```python
from build123d import *

# Parameters (mm, degrees)
SKETCH2_R           = 15
SKETCH2_R_2         = 3
SKETCH2_R_3         = 2.3
BOSS_EXTRUDE1_DEPTH = 4
SKETCH3_R           = 17
SKETCH3_R_2         = 1.475
SKETCH3_R_3         = 1
BOSS_EXTRUDE2_DEPTH = 3
SKETCH8_R           = 15
SKETCH8_R_2         = 12.3
BOSS_EXTRUDE5_DEPTH = 3


with BuildPart() as part:
    # Sketch2 → Boss-Extrude1 (new body)
    with BuildSketch(Plane.XY):
        Circle(SKETCH2_R)
        Circle(SKETCH2_R_2, mode=Mode.SUBTRACT)
        with Locations((-8, 0)):
            Circle(SKETCH2_R_3, mode=Mode.SUBTRACT)
        with Locations((0, 8)):
            Circle(SKETCH2_R_3, mode=Mode.SUBTRACT)
        with Locations((8, 0)):
            Circle(SKETCH2_R_3, mode=Mode.SUBTRACT)
        with Locations((0, -8)):
            Circle(SKETCH2_R_3, mode=Mode.SUBTRACT)
    extrude(amount=BOSS_EXTRUDE1_DEPTH)

    # Sketch3 → Boss-Extrude2 (add)
    with BuildSketch(Plane.XY):
        Circle(SKETCH3_R)
        Circle(SKETCH3_R_2, mode=Mode.SUBTRACT)
        with Locations((-15.8, 0)):
            Circle(SKETCH3_R_3, mode=Mode.SUBTRACT)
        with Locations((15.8, 0)):
            Circle(SKETCH3_R_3, mode=Mode.SUBTRACT)
    extrude(amount=-BOSS_EXTRUDE2_DEPTH)

    # Sketch7 → Cut-Revolve1 (revolve, cut)
    with BuildSketch(Plane(origin=(0, 0, 0), x_dir=(0, 0, -1), z_dir=(1, 0, 0))):
        with BuildLine():
            Line((-4, 15), (0, 15))
            ThreePointArc((0, 15), (-2, 13.505217823), (-4, 15))
        make_face()
    revolve(axis=Axis((0, 0, 0), (0, 0, 1)), mode=Mode.SUBTRACT)

    # Sketch8 → Boss-Extrude5 (add)
    with BuildSketch(Plane.XY.offset(4)):
        Circle(SKETCH8_R)
        Circle(SKETCH8_R_2, mode=Mode.SUBTRACT)
    extrude(amount=BOSS_EXTRUDE5_DEPTH)


solid = part.part
```
Input: part model. Units: mm. Frame: model coordinates. A direction names the side the tool comes from. Give positions to 0.01 mm unless a question says otherwise; leave off trailing zeros. Order: outer loops, then holes, each group sorted by start corner. A loop starts at its lowest first (then second) coordinate and runs counter-clockwise, first axis right, second up. Notation, with made-up numbers: M -16.75,61.25 L 12.25,61.25 A11 cw 12.25,75.25 Z; hole C 36.25,65.25 d2. An arc over 180 degrees is marked long. One line per question, with ' | ' between items.
1) Section D-D on z = 4.75. Output: boundary loops of the cut face in (x, y).
Filled in:
outline: C 0,0 d30; hole C 0,0 d24.6
2) Section C-C on y = 0. State how many separate pieces and enclosed holes the cut face has, and give its area (3 significant figures).
Filled in:
separate pieces: 4 | enclosed holes: 0 | area: 148 mm2
3) Ray query, L1, parallel to Z at x = 4, y = -4; L2, parallel to Z at x = 12, y = -10; L3, parallel to X at y = 2.5, z = 5.75. Return the intervals inside material, ascending.
Filled in:
L1: z = -3 to 4 | L2: z = -3 to 0 | L3: x = -14.79 to -12.04, 12.04 to 14.79
4) Section B-B on z = -1.5. Output: boundary loops of the cut face in (x, y) (3 decimals).
Filled in:
outline: C 0,0 d34; hole C -15.8,0 d2; hole C 0,0 d2.95; hole C 15.8,0 d2
5) Draft query along Y for faces 4 (the face through (-0.3, -5.72, 1.97)), 5 (the face through (9.139, 14.334, -1.479)), 6 (the face through (9, -13, 0)). Return one class per face: pulls with the +Y half, pulls with the -Y half, needs draft (parallel to the pull), parting line crosses it, or undercut.
Filled in:
face 4: undercut | face 5: parting line crosses it | face 6: needs draft
6) Contact query for flat-ended pins moving along their axis: P1, Ø2.5, axis at x = 0, y = 9, coming from the +Z side; P2, Ø6, axis at x = -10.5, z = 5, coming from the +Y side; P3, Ø2.5, axis at x = 0, y = 0, coming from the -Z side; P4, Ø2, axis at y = 11, z = 2.5, coming from the +X side. Output: stop coordinate, or through.
Filled in:
P1: stops at z = 0 | P2: stops at y = 12.99 | P3: passes through | P4: stops at x = 9.33
7) Access query for faces 1 (the face through (8, 0, 0)), 2 (the face through (-2.3, 12.3, 7)), 3 (the face through (-16.8, 0, -1.5)). Directions: +Z, -Z, +X, -X, +Y, -Y. A direction counts if a zero-diameter tool reaches every point of the face in a straight line with its end or side. Return the directions, or none.
Filled in:
face 1: +Z | face 2: +Z, +X, -X, +Y, -Y | face 3: -Z
